```python
from build123d import *

# Parameters (mm, degrees)
SKETCH2_R           = 1.25
BOSS_EXTRUDE1_DEPTH = 8
BOSS_EXTRUDE2_DEPTH = 7
SKETCH3_R           = 0.15
CUT_EXTRUDE1_DEPTH  = 21.967832506
CUT_EXTRUDE2_START  = -6
SKETCH4_R           = 1.25
CUT_EXTRUDE2_DEPTH  = 6


with BuildPart() as part:
    # Sketch2 → Boss-Extrude1 (new body)
    with BuildSketch(Plane.YZ):
        with BuildLine():
            ThreePointArc((-4.35, -14.45), (-3.075914484, -17.525914513), (4.1e-08, -18.8))
            ThreePointArc((4.1e-08, -18.8), (3.075914513, -17.525914484), (4.35, -14.45))
            Line((4.35, -14.45), (6.1, 0))
            Line((6.1, 0), (6.1, 0.55))
            ThreePointArc((6.1, 0.55), (6.070921356, 1.144906627), (5.983962658, 1.734141424))
            Line((5.983962658, 1.734141424), (3.25, 15.55))
            ThreePointArc((3.25, 15.55), (2.298097039, 17.848097039), (0, 18.8))
            ThreePointArc((0, 18.8), (-2.298097039, 17.848097039), (-3.25, 15.55))
            Line((-3.25, 15.55), (-5.983962658, 1.734141424))
            ThreePointArc((-5.983962658, 1.734141424), (-6.070921356, 1.144906627), (-6.1, 0.55))
            Line((-6.1, 0.55), (-6.1, 0))
            Line((-6.1, 0), (-4.35, -14.45))
        make_face()
        with BuildLine():
            Line((3.550344828, -0.045862069), (2.35, -14.45))
            ThreePointArc((2.35, -14.45), (0, -16.8), (-2.35, -14.45))
            Line((-2.35, -14.45), (-3.550344828, -0.045862069))
            ThreePointArc((-3.550344828, -0.045862069), (-3.58756473, 0.251036273), (-3.6, 0.55))
            ThreePointArc((-3.6, 0.55), (0, 4.15), (3.6, 0.55))
            ThreePointArc((3.6, 0.55), (3.58756473, 0.251036273), (3.550344828, -0.045862069))
        make_face(mode=Mode.SUBTRACT)
        with Locations(Location((0, 15.55, 0), (0, 0, 270))):
            Circle(SKETCH2_R, mode=Mode.SUBTRACT)
    extrude(amount=BOSS_EXTRUDE1_DEPTH)

    # Sketch2_3 → Boss-Extrude2 (add)
    with BuildSketch(Plane.YZ):
        with BuildLine():
            ThreePointArc((-2.35, -14.45), (0, -16.8), (2.35, -14.45))
            Line((2.35, -14.45), (3.550344828, -0.045862069))
            Line((3.550344828, -0.045862069), (3.6, 0.55))
            ThreePointArc((3.6, 0.55), (0, 4.15), (-3.6, 0.55))
            Line((-3.6, 0.55), (-3.550344828, -0.045862069))
            Line((-3.550344828, -0.045862069), (-2.35, -14.45))
        make_face()
    extrude(amount=BOSS_EXTRUDE2_DEPTH)

    # Sketch3 → Cut-Extrude1 (cut, through all)
    with BuildSketch(Plane.YZ.offset(7)):
        with Locations(Location((0, 0.55, 0), (0, 0, 270))):
            Circle(SKETCH3_R)
        with Locations(Location((0, -14.45, 0), (0, 0, 270))):
            Circle(SKETCH3_R)
    extrude(amount=-CUT_EXTRUDE1_DEPTH, mode=Mode.SUBTRACT)

    # Sketch4 → Cut-Extrude2 (cut)
    with BuildSketch(Plane.YZ.offset(8).offset(CUT_EXTRUDE2_START)):
        with BuildLine():
            Line((-5.209069729, 5.65), (5.209069729, 5.65))
            Line((5.209069729, 5.65), (3.25, 15.55))
            ThreePointArc((3.25, 15.55), (0, 18.8), (-3.25, 15.55))
            Line((-3.25, 15.55), (-5.209069729, 5.65))
        make_face()
        with Locations(Location((0, 15.55, 0), (0, 0, 270))):
            Circle(SKETCH4_R, mode=Mode.SUBTRACT)
    extrude(amount=CUT_EXTRUDE2_DEPTH, mode=Mode.SUBTRACT)


solid = part.part
```
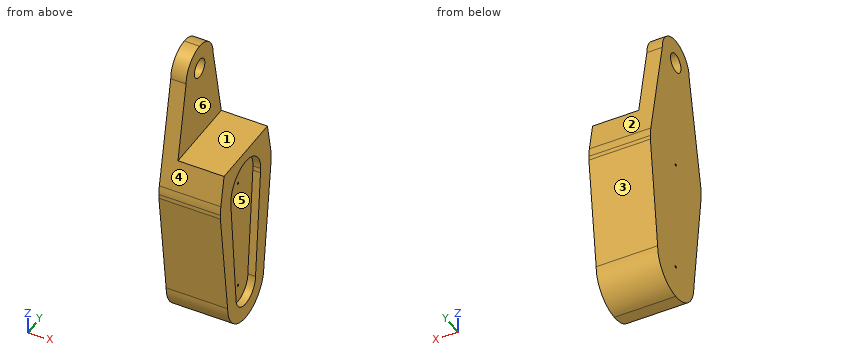
Build history of the part. All positions in model axes, mm. Face numbers are marked on the shaded views. A direction names the side the tool comes from. Give positions to 0.01 mm unless a question says otherwise; leave off trailing zeros. Loops run counter-clockwise (first coordinate to the right, second up) from the corner with the lowest first, then second, coordinate; pieces in that order, holes last. Notation, with made-up numbers: (-30.75, 86.5) - (0.25, 86.5) arc R35 ccw to (0.25, 122.5) - close; hole circle Ø11 at (22, -25). An arc over 180 degrees is marked (long way). Use a Markdown table: item, result.
(1) Wall check: line 1 along Y through (x, z) = (2, -14.45); line 2 along Z through (x, y) = (3, 0.25); line 3 along Y through (x, z) = (2, -1). Give the ranges that are in metal, low to high.
Taken from the geometry:
| item | result |
|---|---|
| line 1 | -4.35 to -0.15, 0.15 to 4.35 |
| line 2 | -18.79 to 5.65 |
| line 3 | -5.98 to 5.98 |
(2) Band-saw the part on D-D (y = 4). Give the cut face in (x, z).
Taken from the geometry:
| item | result |
|---|---|
| outline | (0, -16.16) - (8, -16.16) - (8, 5.65) - (2, 5.65) - (2, 11.76) - (0, 11.76) - close |
(3) Band-saw the part on C-C (z = -11.5). Give the cut face in (x, y).
Taken from the geometry:
| item | result |
|---|---|
| outline | (0, -4.71) - (8, -4.71) - (8, -2.6) - (7, -2.6) - (7, 2.6) - (8, 2.6) - (8, 4.71) - (0, 4.71) - close |
(4) Band-saw the part on A-A (x = 5.5). Give the cut face in (y, z).
Taken from the geometry:
| item | result |
|---|---|
| outline | (-6.1, 0) - (-4.35, -14.45) arc R4.35 ccw to (4.35, -14.45) - (6.1, 0) - (6.1, 0.55) arc R6.1 ccw to (5.98, 1.73) - (5.21, 5.65) - (-5.21, 5.65) - (-5.98, 1.73) arc R6.1 ccw to (-6.1, 0.55) - close; hole (-3.6, 0.55) arc R3.6 ccw to (-3.55, -0.05) - close; hole circle Ø0.3 at (0, -14.45); hole circle Ø0.3 at (0, 0.55); hole (3.55, -0.05) arc R3.6 ccw to (3.6, 0.55) - close |
(5) Pull direction Z, two halves, no side cores. Call the marked faces 3, 4, 5 and 6: +Z half, -Z half, draft (parallel to the pull), parting line (faces both ways), or undercut.
Taken from the geometry:
| item | result |
|---|---|
| face 3 | -Z half |
| face 4 | +Z half |
| face 5 | undercut |
| face 6 | draft |
(6) Which spindle directions (+Z, -Z, +X, -X, +Y, -Y) get a long thin tool onto all of the face, cutting with end or side? Do the marked faces 1 and 2. Say none if no direction does.
Taken from the geometry:
| item | result |
|---|---|
| face 1 | +Z, +X, +Y, -Y |
| face 2 | +Z, +X, -X, +Y |
(7) Drop flat-ended pins along their axis: pin 1 Ø2 at (y, z) = (0, 15.55) entering from +X; pin 2 Ø3.5 at (y, z) = (1.5, -2) entering from +X; pin 3 Ø1 at (x, y) = (5, -4) entering from +Z; pin 4 Ø1 at (x, y) = (7, -3.5) entering from -Z. Give the stop position or say it passes through.
Taken from the geometry:
| item | result |
|---|---|
| pin 1 | through |
| pin 2 | x = 7 |
| pin 3 | z = 5.65 |
| pin 4 | z = -17.6 |
(8) Band-saw the part on B-B (y = 0.75). Give the cut face in (x, z), and give its area (3 significant figures).
Taken from the geometry:
| item | result |
|---|---|
| outline | (0, -18.73) - (8, -18.73) - (8, -16.68) - (7, -16.68) - (7, 4.07) - (8, 4.07) - (8, 5.65) - (2, 5.65) - (2, 14.55) - (0, 14.55) - close; (0, 16.55) - (2, 16.55) - (2, 18.71) - (0, 18.71) - close |
| area | 196 mm2 |
